Verification items for the finished model (mm, model axes). A direction names the side the tool comes from. Coordinates: 2 decimals unless noted, no trailing zeros. Order: outer loops, then holes, each group sorted by start corner. A loop starts at its lowest first (then second) coordinate and runs counter-clockwise, first axis right, second up.
Q1. Cross-section at A-A, the plane y = 23.57. Record the boundary of the cut face in (x, z), and give its area (3 significant figures).
Q2. Cross-section at D-D, the plane x = 23.57. Record the boundary of the cut face in (y, z), and give its area (3 significant figures).
Q3. Depth check by flat-ended pin: P1, Ø1.5, axis at x = 22, z = 5, coming from the +Y side; P2, Ø1.5, axis at y = 84, z = 4, coming from the +X side. Enter the tip coordinate at first touch or a pass-through.
Q4. Thickness scan on line 1 (Y direction, x = 23.57, z = 4.5); line 2 (X direction, y = 21.5, z = 4.2); line 3 (X direction, y = -20, z = 0.65). Record the ranges inside material, lowest first.
Q5. Draft check along Y on faces 1 (the flat face through (44, -30, 3)), 2 (the cylindrical face through (6.867, 32.625, 2.958)), 3 (the cylindrical face through (99.248, 95.755, 2.958)). Enter one of: pulls with the +Y half, pulls with the -Y half, needs draft (parallel to the pull), parting line crosses it, or undercut.
Q6. Cross-section at C-C, the plane z = 5.05. Count the separate pieces of the cut face and the enclosed holes in it, and give its area (3 significant figures).
Q7. Cross-section at B-B, the plane x = 91.5. Record the boundary of the cut face in (y, z).
Q8. Set-up check for faces 4 (the cylindrical face through (54.62, -21.89, 3.04)), 5 (the flat face through (56, 52, 3)): record each of +Z, -Z, +X, -X, +Y, -Y from which the full face is reachable in a straight line by a thin tool's end or side.
from build123d import *

# Parameters (mm, degrees)
SKETCH1_W           = 60
SKETCH1_H           = 60
SKETCH1_R           = 4
SKETCH1_R_2         = 26
BOSS_EXTRUDE1_DEPTH = 10
FILLET1_R           = 5
SKETCH3_R           = 26
SKETCH3_R_2         = 24
BOSS_EXTRUDE2_DEPTH = 3
SKETCH4_R           = 20
CUT_EXTRUDE1_DEPTH  = 1.6
SKETCH5_R           = 8
CUT_EXTRUDE2_DEPTH  = 158.213840184
SKETCH6_R           = 2.5
CUT_EXTRUDE3_DEPTH  = 158.307442752
SKETCH8_R           = 12
CUT_EXTRUDE5_DEPTH  = 158.213840184
SKETCH9_R           = 12
CUT_EXTRUDE6_DEPTH  = 4
SKETCH10_R          = 1.5
CUT_EXTRUDE7_DEPTH  = 158.103887747
SKETCH11_R          = 1.55
CUT_EXTRUDE8_DEPTH  = 158.103887747
SKETCH12_R          = 1.5
BOSS_EXTRUDE3_DEPTH = 6
SKETCH13_R          = 2.55
CUT_EXTRUDE9_DEPTH  = 158.103887747


with BuildPart() as part:
    # Sketch1 → Boss-Extrude1 (new body)
    # profile 1 of 3: a face of its own
    with BuildSketch(Plane.XY):
        with BuildLine():
            Line((52.853069415, 91.422204295), (-30, 30))
            Line((-30, 30), (30, 30))
            Line((30, 30), (30, -30))
            Line((30, -30), (120.187635495, -30))
            Line((120.187635495, -30), (120.187635495, 59.997840668))
            ThreePointArc((120.187635495, 59.997840668), (61.848621816, 22.844663083), (52.853069415, 91.422204295))
        make_face()
    # profile 2 of 3: a face of its own
    with BuildSketch(Plane.XY):
        Rectangle(SKETCH1_W, SKETCH1_H)
        Circle(SKETCH1_R, mode=Mode.SUBTRACT)
    # profile 3 of 3: a face of its own
    with BuildSketch(Plane.XY):
        with BuildLine():
            Line((56.774720343, 94.329476725), (52.853069415, 91.422204295))
            ThreePointArc((52.853069415, 91.422204295), (61.848621816, 22.844663083), (120.187635495, 59.997840668))
            ThreePointArc((120.187635495, 59.997840668), (98.707759454, 96.052864736), (56.774720343, 94.329476725))
        make_face()
        with Locations((79.187635495, 59.997840668)):
            Circle(SKETCH1_R_2, mode=Mode.SUBTRACT)
    extrude(amount=BOSS_EXTRUDE1_DEPTH)

    # Fillet1
    fillet1_edges = [part.edges().sort_by_distance(p)[0] for p in [
        (120.187635495, -30, 5),
        (-30, -30, 5),
        (-30, 30, 5),
    ]]
    fillet(fillet1_edges, radius=FILLET1_R)

    # Sketch3 → Boss-Extrude2 (add)
    with BuildSketch(Plane(origin=(0, 0, 0), x_dir=(-1, 0, 0), z_dir=(0, 0, -1))):
        with Locations((-79.187635495, 59.997840668)):
            Circle(SKETCH3_R)
        with Locations((-79.187635495, 59.997840668)):
            Circle(SKETCH3_R_2, mode=Mode.SUBTRACT)
    extrude(amount=-BOSS_EXTRUDE2_DEPTH)

    # Sketch4 → Cut-Extrude1 (cut)
    with BuildSketch(Plane.XY.offset(10)):
        Circle(SKETCH4_R)
    extrude(amount=-CUT_EXTRUDE1_DEPTH, mode=Mode.SUBTRACT)

    # Sketch5 → Cut-Extrude2 (cut, through all)
    with BuildSketch(Plane.XY.offset(8.4)):
        Circle(SKETCH5_R)
    extrude(amount=-CUT_EXTRUDE2_DEPTH, mode=Mode.SUBTRACT)

    # Sketch6 → Cut-Extrude3 (cut, through all)
    with BuildSketch(Plane.XY.offset(10)):
        with Locations((23.57, 23.57)):
            Circle(SKETCH6_R)
        with Locations((-23.57, 23.57)):
            Circle(SKETCH6_R)
        with Locations((-23.57, -23.57)):
            Circle(SKETCH6_R)
        with Locations((23.57, -23.57)):
            Circle(SKETCH6_R)
    extrude(amount=-CUT_EXTRUDE3_DEPTH, mode=Mode.SUBTRACT)

    # Sketch8 → Cut-Extrude5 (cut, through all)
    with BuildSketch(Plane.XY.offset(8.4)):
        Circle(SKETCH8_R)
    extrude(amount=-CUT_EXTRUDE5_DEPTH, mode=Mode.SUBTRACT)

    # Sketch9 → Cut-Extrude6 (cut)
    with BuildSketch(Plane.XY.offset(10)):
        with BuildLine():
            Line((-25, -30), (115.187635495, -30))
            ThreePointArc((115.187635495, -30), (118.723169401, -28.535533906), (120.187635495, -25))
            Line((120.187635495, -25), (120.187635495, 59.997840668))
            ThreePointArc((120.187635495, 59.997840668), (98.707759454, 96.052864736), (56.774720343, 94.329476725))
            Line((56.774720343, 94.329476725), (-27.977688922, 31.499217893))
            ThreePointArc((-27.977688922, 31.499217893), (-29.465895465, 29.731087062), (-30, 27.482581404))
            Line((-30, 27.482581404), (-30, -25))
            ThreePointArc((-30, -25), (-28.535533906, -28.535533906), (-25, -30))
        make_face()
        Circle(SKETCH9_R, mode=Mode.SUBTRACT)
    extrude(amount=-CUT_EXTRUDE6_DEPTH, mode=Mode.SUBTRACT)

    # Sketch10 → Cut-Extrude7 (cut, through all)
    with BuildSketch(Plane.XY.offset(6)):
        with Locations((53.187635495, -16.002159332)):
            Circle(SKETCH10_R)
        with Locations((105.187635495, -16.002159332)):
            Circle(SKETCH10_R)
        with Locations((105.187635495, 13.997840668)):
            Circle(SKETCH10_R)
        with Locations((79.187635495, -1.002159332)):
            Circle(SKETCH10_R)
        with Locations((53.187635495, 13.997840668)):
            Circle(SKETCH10_R)
        with Locations((79.187635495, 13.997840668)):
            Circle(SKETCH10_R)
    extrude(amount=-CUT_EXTRUDE7_DEPTH, mode=Mode.SUBTRACT)

    # Sketch11 → Cut-Extrude8 (cut, through all)
    with BuildSketch(Plane.XY.offset(6)):
        with Locations((53.187635495, -21.3)):
            Circle(SKETCH11_R)
        with Locations((105.187635495, -21.3)):
            Circle(SKETCH11_R)
    extrude(amount=-CUT_EXTRUDE8_DEPTH, mode=Mode.SUBTRACT)

    # Sketch12 → Boss-Extrude3 (add)
    with BuildSketch(Plane.XY.offset(6)):
        with Locations((53.187635495, -16.002159332)):
            Circle(SKETCH12_R)
        with Locations((105.187635495, -16.002159332)):
            Circle(SKETCH12_R)
    extrude(amount=-BOSS_EXTRUDE3_DEPTH)

    # Sketch13 → Cut-Extrude9 (cut, through all)
    with BuildSketch(Plane(origin=(0, 0, 0), x_dir=(-1, 0, 0), z_dir=(0, 0, -1))):
        with Locations((-8.043910978, 34.887394427)):
            Circle(SKETCH13_R)
    extrude(amount=-CUT_EXTRUDE9_DEPTH, mode=Mode.SUBTRACT)


solid = part.part
Check values:
1. outline: (-30, 0) - (-26.07, 0) - (-26.07, 6) - (-30, 6) - close; (-21.07, 0) - (21.07, 0) - (21.07, 6) - (-21.07, 6) - close; (26.07, 0) - (120.19, 0) - (120.19, 6) - (26.07, 6) - close
1. area: 841 mm2
2. outline: (-30, 0) - (-26.07, 0) - (-26.07, 6) - (-30, 6) - close; (-21.07, 0) - (21.07, 0) - (21.07, 6) - (-21.07, 6) - close; (26.07, 0) - (69.71, 0) - (69.71, 6) - (26.07, 6) - close
2. area: 538 mm2
3. P1: stops at y = 69.11
3. P2: stops at x = 112.96
4. line 1: y = -30 to -26.07, -21.07 to 21.07, 26.07 to 69.71
4. line 2: x = -30 to -24.97, -22.17 to 22.17, 24.97 to 120.19
4. line 3: x = -30 to 52.34, 54.03 to 104.34, 106.03 to 120.19
5. face 1: pulls with the -Y half
5. face 2: undercut
5. face 3: pulls with the +Y half
6. separate pieces: 1
6. enclosed holes: 13
6. area: 13,200 mm2
7. outline: (-30, 0) - (39.4, 0) - (39.4, 3) - (37.1, 3) - (37.1, 6) - (-30, 6) - close; (80.6, 0) - (99.11, 0) - (99.11, 6) - (82.9, 6) - (82.9, 3) - (80.6, 3) - close
8. face 4: +Z, -Z
8. face 5: +Z
